Geometry check sheet. Reference: the model listing, model coordinates, mm. A direction names the side the tool comes from. Give positions to 0.01 mm unless a question says otherwise; leave off trailing zeros. Loops run counter-clockwise (first coordinate to the right, second up) from the corner with the lowest first, then second, coordinate; pieces in that order, holes last. Notation, with made-up numbers: (7.25, -23) -> (58.25, -23) arc R17 ccw to (58.25, 8) -> close; hole circle Ø5 at (26.25, 49). An arc over 180 degrees is marked (long way). Answer as a JSON object with one key per item and string values.
from build123d import *

# Parameters (mm, degrees)
F0_R     = 11
F1_DEPTH = 3
F2_R     = 2
F3_R     = 7.5
F4_DEPTH = 2
F5_R     = 4
F5_R_2   = 2.5
F6_DEPTH = 7


with BuildPart() as f1:
    # F0 (on Top) → F1 (new body)
    with BuildSketch(Plane.XY):
        Circle(F0_R)
    extrude(amount=F1_DEPTH)

    # F2
    f2_edges = [f1.edges().sort_by_distance(p)[0] for p in [
        (-11, 0, 0),
    ]]
    fillet(f2_edges, radius=F2_R)

    # F3 (on face) → F4 (join)
    with BuildSketch(Plane.XY.offset(3)):
        Circle(F3_R)
    extrude(amount=F4_DEPTH)

    # F5 (on face) → F6 (join)
    with BuildSketch(Plane.XY.offset(5)):
        Circle(F5_R)
        Circle(F5_R_2, mode=Mode.SUBTRACT)
    extrude(amount=F6_DEPTH)


solid = f1.part
1) Section check C-C on z = 11.25. Record the cut outline in (x, y), plus the area to 3 significant figures.
Geometry check:
{"outline": "circle Ø8 at (0, 0); hole circle Ø5 at (0, 0)", "area": "30.6 mm2"}
2) Tool access check on faces 4 (the face through (2, 2, 12)), 5 (the face through (-0.54, -2.44, 8.45)). Record the directions out of +Z, -Z, +X, -X, +Y, -Y that give a thin tool (end or side, any length) a straight path to the whole face; none if there is none.
Geometry check:
{"face 4": "+Z, +X, -X, +Y, -Y", "face 5": "+Z"}
3) Draft check along X on faces 1 (the face through (0, 0, 5)), 2 (the face through (-0.867, -3.905, 8.451)), 3 (the face through (0, 0, 0)). Enter one of: pulls with the +X half, pulls with the -X half, needs draft (parallel to the pull), parting line crosses it, or undercut.
Geometry check:
{"face 1": "undercut", "face 2": "parting line crosses it", "face 3": "needs draft"}
4) Depth check by flat-ended pin: P1, Ø5, axis at x = -6, z = 5, coming from the +Y side; P2, Ø6, axis at x = -3, z = 6.5, coming from the -Y side. Enter the tip coordinate at first touch or a pass-through.
Geometry check:
{"P1": "stops at y = 10.04", "P2": "stops at y = -7.49"}
5) Section check A-A on x = 0. Record the cut outline in (y, z), plus the area to 3 significant figures.
Geometry check:
{"outline": "(-11, 2) arc R2 ccw to (-9, 0) -> (9, 0) arc R2 ccw to (11, 2) -> (11, 3) -> (7.5, 3) -> (7.5, 5) -> (4, 5) -> (4, 12) -> (2.5, 12) -> (2.5, 5) -> (-2.5, 5) -> (-2.5, 12) -> (-4, 12) -> (-4, 5) -> (-7.5, 5) -> (-7.5, 3) -> (-11, 3) -> close", "area": "115 mm2"}
6) Material ranges on line 1 along Y through (x, z) = (0, 7.75); line 2 along Z through (x, y) = (-1, 2); line 3 along Z through (x, y) = (8.25, 3), recorded low to high. Write a range as from..to.
Geometry check:
{"line 1": "y = -4..-2.5, 2.5..4", "line 2": "z = 0..5", "line 3": "z = 0..3"}
